Build history of the part. All positions in model axes, mm. A direction names the side the tool comes from. Round coordinates to 2 decimals unless told otherwise and drop trailing zeros. Loops run counter-clockwise (first coordinate to the right, second up) from the corner with the lowest first, then second, coordinate; pieces in that order, holes last. Notation, with made-up numbers: (61.25, -33) - (66.25, -33) arc R17 cw to (66.25, -26) - close; hole circle Ø5 at (54.5, -5.5). An arc over 180 degrees is marked (long way). Use a Markdown table: item, result.
Autodesk Inventor part; units mm, degrees
ref_plane "YZ Plane" through (0, 0, 0) normal (1, 0, 0) x (0, 1, 0)
ref_plane "XZ Plane" through (0, 0, 0) normal (0, 1, 0) x (-1, 0, 0)
ref_plane "XY Plane" through (0, 0, 0) normal (0, 0, 1) x (1, 0, 0)
sketch "Sketch1" plane through (0, 0, 0) normal (0, 0, 1) x (1, 0, 0)
  line L0 (0, 0) -> (200, 0)
  line L1 (200, 0) -> (200, 300)
  line L2 (200, 300) -> (0, 300)
  line L3 (0, 300) -> (0, 0)
  dimension "d0" = 200
  dimension "d1" = 300
extrude "Extrusion1" add sketch "Sketch1" along normal blind 10
sketch "Sketch2" plane through (0, 0, 10) normal (0, 0, 1) x (1, 0, 0)
  circle A0 centre (5, 195) radius 2.4585
  line L0 (0, 300) -> (0, 0)
  circle A1 centre (5, 260) radius 2.4585
  circle A2 centre (195, 260) radius 2.4585
  circle A3 centre (195, 195) radius 2.4585
hole "Hole1" at (195, 195, 10) at (195, 260, 10) at (5, 195, 10) at (5, 260, 10) direction (0, 0, -1) diameter 7 end through all counterbore diameter 11 counterbore depth 5
sketch "Sketch3" plane through (0, 0, 10) normal (0, 0, 1) x (1, 0, 0)
  circle A0 centre (24, 150) radius 2.4585
  circle A1 centre (24, 150) radius 2.4585
  circle A2 centre (56, 150) radius 2.4585
  circle A3 centre (144, 150) radius 2.4585
  circle A4 centre (176, 150) radius 2.4585
  point P0 (0, 0)
hole "Hole2" at (176, 150, 10) at (144, 150, 10) at (56, 150, 10) at (24, 150, 10) direction (0, 0, -1) diameter 7 end through all counterbore diameter 11 counterbore depth 5
sketch "Sketch4" plane through (0, 0, 0) normal (0, 0, -1) x (-1, 0, 0)
  circle A0 centre (-70, 195) radius 3
  circle A1 centre (-130, 195) radius 3
  line L0 (0, 300) -> (0, 0)
  line L1 (-200, 0) -> (-200, 300)
  circle A2 centre (-70, 260) radius 3
  circle A3 centre (-130, 260) radius 3
  circle A4 centre (-70, 40) radius 3
  circle A5 centre (-130, 40) radius 3
  circle A6 centre (-70, 105) radius 3
  circle A7 centre (-130, 105) radius 3
  line L2 (0, 0) -> (-200, 0)
  dimension "d18" = 6
  dimension "d19" = 70
  dimension "d20" = 70
  dimension "d21" = 6
  dimension "d22" = 6
  dimension "d23" = 6
  dimension "d24" = 40
  dimension "d25" = 40
  dimension "d26" = 65
  dimension "d27" = 65
hole "Hole3" at (130, 195, 0) at (130, 260, 0) at (70, 260, 0) at (70, 195, 0) at (70, 105, 0) at (130, 105, 0) at (130, 40, 0) at (70, 40, 0) direction (0, 0, 1) diameter 7 end through all counterbore diameter 11 counterbore depth 5
properties part number "200x300(10li)"
Q1. Cut at A-A, the plane x = 24. List the corners of the cut face in (y, z), plus the area to 3 significant figures.
Results found:
| item | result |
|---|---|
| outline | (0, 0) - (146.5, 0) - (146.5, 5) - (144.5, 5) - (144.5, 10) - (0, 10) - close; (153.5, 0) - (300, 0) - (300, 10) - (155.5, 10) - (155.5, 5) - (153.5, 5) - close |
| area | 2,910 mm2 |
Q2. Pull direction X, two halves, no side cores. Call faces 1 (the face through (3.95, 191.66, 2.46)), 2 (the face through (200, 148, 5)), 3 (the face through (189.504, 194.791, 7.465)), 4 (the face through (99, 152, 10)): pulls with the +X half, pulls with the -X half, needs draft (parallel to the pull), parting line crosses it, or undercut.
Results found:
| item | result |
|---|---|
| face 1 | undercut |
| face 2 | pulls with the +X half |
| face 3 | undercut |
| face 4 | needs draft |
Q3. Which spindle directions (+Z, -Z, +X, -X, +Y, -Y) get a long thin tool onto all of the face, cutting with end or side? Do faces 5 (the face through (130, 109, 5)), 6 (the face through (148, 150, 5)), 7 (the face through (145.341, 146.767, 2.465)). Say none if no direction does.
Results found:
| item | result |
|---|---|
| face 5 | -Z |
| face 6 | +Z |
| face 7 | +Z, -Z |
Q4. Drop flat-ended pins along their axis: pin 1 (9 mm diameter, centred on x = 176, y = 149.5, fed in from +Z); pin 2 (5.5 mm diameter, centred on x = 71, y = 257.5, fed in from -Z); pin 3 (5.5 mm diameter, centred on x = 70, y = 105, fed in from +Z). Give the stop position or say it passes through.
Results found:
| item | result |
|---|---|
| pin 1 | stops at z = 5 |
| pin 2 | stops at z = 5 |
| pin 3 | passes through |
Q5. Probe line 1 (X direction, y = 260, z = 6.45); line 2 (X direction, y = 150, z = 3.25); line 3 (X direction, y = 40, z = 6.95). List the from-to ranges inside material, lowest first.
Results found:
| item | result |
|---|---|
| line 1 | x = 10.5 to 66.5, 73.5 to 126.5, 133.5 to 189.5 |
| line 2 | x = 0 to 20.5, 27.5 to 52.5, 59.5 to 140.5, 147.5 to 172.5, 179.5 to 200 |
| line 3 | x = 0 to 66.5, 73.5 to 126.5, 133.5 to 200 |
Q6. Cut at C-C, the plane z = 6.5. Count the separate pieces of the cut face and the enclosed holes in it, plus the area to 3 significant figures.
Results found:
| item | result |
|---|---|
| separate pieces | 1 |
| enclosed holes | 12 |
| area | 58,900 mm2 |
Q7. Cut at B-B, the plane y = 105. List the corners of the cut face in (x, z), plus the area to 3 significant figures.
Results found:
| item | result |
|---|---|
| outline | (0, 0) - (64.5, 0) - (64.5, 5) - (66.5, 5) - (66.5, 10) - (0, 10) - close; (73.5, 5) - (75.5, 5) - (75.5, 0) - (124.5, 0) - (124.5, 5) - (126.5, 5) - (126.5, 10) - (73.5, 10) - close; (133.5, 5) - (135.5, 5) - (135.5, 0) - (200, 0) - (200, 10) - (133.5, 10) - close |
| area | 1,820 mm2 |
